The listing builds one solid part. Answer for the finished solid, in the listing's coordinates (mm). A direction names the side the tool comes from. Coordinates: 2 decimals unless noted, no trailing zeros. Write each loop counter-clockwise with the first axis right and the second up, starting at its lowest first coordinate (ties: lowest second). Pieces come first, ordered by that corner, then holes.
```python
from build123d import *

# Parameters (mm, degrees)
SKETCH_R              = 138.5
SKETCH_R_2            = 128.5
PAD_DEPTH             = 30
SKETCH002_R           = 1
POCKET001_DEPTH       = 28
SKETCH003_R           = 143.5
SKETCH003_R_2         = 136.5
PAD001_DEPTH          = 15
POCKET002_DEPTH       = 30
POLARPATTERN002_COUNT = 6


with BuildPart() as part:
    # Sketch → Pad (new body)
    with BuildSketch(Plane.XY):
        Circle(SKETCH_R)
        Circle(SKETCH_R_2, mode=Mode.SUBTRACT)
    extrude(amount=PAD_DEPTH)

    # Sketch002 (on DatumPlane) → Pocket001 (cut)
    with BuildSketch(Plane(origin=(-1, -155, 0), x_dir=(1, 0, 0), z_dir=(0, -1, 0))):
        with Locations((0, 7)):
            Circle(SKETCH002_R)
    extrude(amount=-POCKET001_DEPTH, mode=Mode.SUBTRACT)

    # Sketch003 → Pad001 (join)
    with BuildSketch(Plane.XY):
        with Locations((-0.00298, -0.000479)):
            Circle(SKETCH003_R)
        with Locations((-0.006501, 0.000101)):
            Circle(SKETCH003_R_2, mode=Mode.SUBTRACT)
    extrude(amount=PAD001_DEPTH)

    # Sketch002 (on DatumPlane) → Pocket002 (cut)
    with BuildSketch(Plane(origin=(-1, -155, 0), x_dir=(1, 0, 0), z_dir=(0, -1, 0))):
        with Locations((0, 7)):
            Circle(SKETCH002_R)
    pocket002 = extrude(amount=-POCKET002_DEPTH, mode=Mode.SUBTRACT)

    # PolarPattern002: Pocket002 ×6 about axis
    polarpattern002_axis = Axis((0, 0, 0), (0, 0, 1))
    for i in range(1, POLARPATTERN002_COUNT):
        add(pocket002.rotate(polarpattern002_axis, i * 360 / POLARPATTERN002_COUNT), mode=Mode.SUBTRACT)


solid = part.part
```
(1) Section A-A, the plane x = -53 is taken. Write down the section's boundary in (y, z).
(2) Each of these flat-tipped pins is pushed along its axis until it touches: pin 1 (12 mm diameter, centred on y = -71, z = 13, fed in from +X); pin 2 (10 mm diameter, centred on y = 58.5, z = 17, fed in from -X); pin 3 (3 mm diameter, centred on x = -97, z = 18, fed in from -Y). Where does it stop, or does it pass through?
(3) Find the intervals of material crossed by probe 1 along Z at (x, y) = (-1, -132.25); probe 2 along X at (y, z) = (3, 7.5); probe 3 along Y at (x, z) = (-57.5, 18), in increasing order.
(4) Which of the six approach directions +Z, -Z, +X, -X, +Y, -Y give full straight-line access (tool end or side, diameter ignored) to faces 1 (the cylindrical face through (-27.856, -125.444, 14.79)), 2 (the flat face through (-118, 75, 15))?
(5) For a pull along X with two mould halves and no side action, classify faces 3 (the cylindrical face through (-117.84, 68.09, 7.3)), 4 (the flat face through (-107, -74, 0)), 5 (the cylindrical face through (-113.88, -87.32, 7.4)) as pulls with the +X half, pulls with the -X half, needs draft (parallel to the pull), parting line crosses it, or undercut.
(6) Section B-B, the plane y = -19 is taken. Write down the section's boundary in (x, z), plus the area to 3 significant figures.
Solution:
1. outline: (-133.36, 0) - (-117.06, 0) - (-117.06, 30) - (-127.96, 30) - (-127.96, 15) - (-133.36, 15) - close; (117.06, 0) - (133.35, 0) - (133.35, 15) - (127.96, 15) - (127.96, 30) - (117.06, 30) - close
2. pin 1: stops at x = 127.93
2. pin 2: stops at x = -132.99
2. pin 3: stops at y = -100.31
3. probe 1: z = 0 to 6, 8 to 30
3. probe 2: x = -143.47 to -128.46, 128.46 to 143.47
3. probe 3: y = -126 to -114.92, 114.92 to 126
4. face 1: +Z, -Z
4. face 2: +Z
5. face 3: undercut
5. face 4: needs draft
5. face 5: parting line crosses it
6. outline: (-142.24, 0) - (-127.09, 0) - (-127.09, 30) - (-137.19, 30) - (-137.19, 15) - (-142.24, 15) - close; (127.09, 0) - (142.23, 0) - (142.23, 15) - (137.19, 15) - (137.19, 30) - (127.09, 30) - close
6. area: 758 mm2
